```python
from build123d import *

# Parameters (mm, degrees)
SKETCH1_R           = 75
SKETCH1_R_2         = 1.7
SKETCH1_R_3         = 15
BOSS_EXTRUDE1_DEPTH = 3
SKETCH2_R           = 1.75
CUT_EXTRUDE2_DEPTH  = 107.108435103
SKETCH3_R           = 1.75
CUT_EXTRUDE3_DEPTH  = 107.108435103


with BuildPart() as part:
    # Sketch1 → Boss-Extrude1 (new body)
    with BuildSketch(Plane(origin=(0, 0, 0), x_dir=(1, 0, 0), z_dir=(0, 1, 0))):
        with Locations(Location((0, 0, 0), (0, 0, 270))):
            Circle(SKETCH1_R)
        with Locations(Location((49.497474683, 49.497474683, 0), (0, 0, 270))):
            Circle(SKETCH1_R_2, mode=Mode.SUBTRACT)
        with Locations(Location((-49.497474683, 49.497474683, 0), (0, 0, 270))):
            Circle(SKETCH1_R_2, mode=Mode.SUBTRACT)
        with Locations(Location((-49.497474683, -49.497474683, 0), (0, 0, 270))):
            Circle(SKETCH1_R_2, mode=Mode.SUBTRACT)
        with Locations(Location((49.497474683, -49.497474683, 0), (0, 0, 270))):
            Circle(SKETCH1_R_2, mode=Mode.SUBTRACT)
        with Locations(Location((0, 0, 0), (0, 0, 270))):
            Circle(SKETCH1_R_3, mode=Mode.SUBTRACT)
    extrude(amount=BOSS_EXTRUDE1_DEPTH)

    # Sketch2 → Cut-Extrude2 (cut, through all)
    with BuildSketch(Plane(origin=(0, 0, 0), x_dir=(1, 0, 0), z_dir=(0, 1, 0))):
        with Locations(Location((0, 68.825, 0), (0, 0, 270))):
            Circle(SKETCH2_R)
        with Locations(Location((68.825, 0, 0), (0, 0, 270))):
            Circle(SKETCH2_R)
        with Locations(Location((0, -68.825, 0), (0, 0, 270))):
            Circle(SKETCH2_R)
        with Locations(Location((-68.825, 0, 0), (0, 0, 270))):
            Circle(SKETCH2_R)
    extrude(amount=CUT_EXTRUDE2_DEPTH, mode=Mode.SUBTRACT)

    # Sketch3 → Cut-Extrude3 (cut, through all)
    with BuildSketch(Plane(origin=(0, 0, 0), x_dir=(1, 0, 0), z_dir=(0, 1, 0))):
        with Locations(Location((-43, 25, 0), (0, 0, 270))):
            Circle(SKETCH3_R)
        with Locations(Location((-17, 25, 0), (0, 0, 270))):
            Circle(SKETCH3_R)
        with Locations(Location((-17, -41, 0), (0, 0, 270))):
            Circle(SKETCH3_R)
        with Locations(Location((-43, -41, 0), (0, 0, 270))):
            Circle(SKETCH3_R)
        with Locations(Location((17.505557347, 19.884131141, 0), (0, 0, 270))):
            Circle(SKETCH3_R)
        with Locations(Location((46.494442653, -19.884131141, 0), (0, 0, 270))):
            Circle(SKETCH3_R)
        with Locations(Location((46.494442653, 19.884131141, 0), (0, 0, 270))):
            Circle(SKETCH3_R)
        with Locations(Location((17.505557347, -19.884131141, 0), (0, 0, 270))):
            Circle(SKETCH3_R)
        Polygon((31.243092686, 49.296238796), (12.765502036, 56.949907443), (14.678919198, 61.569305106), (33.156509848, 53.915636458), align=None)
    extrude(amount=CUT_EXTRUDE3_DEPTH, mode=Mode.SUBTRACT)


solid = part.part
```
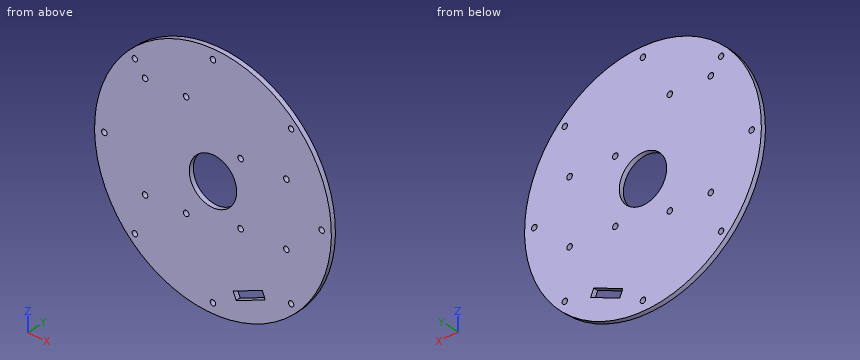
Source: CAD feature listing. Evaluate the final solid. Frame: model axes, mm. Give positions to 0.01 mm unless a question says otherwise; leave off trailing zeros. Write each loop counter-clockwise with the first axis right and the second up, starting at its lowest first coordinate (ties: lowest second). Pieces come first, ordered by that corner, then holes.
1. Section query D-D (z = 0). Return the cut outline in (x, y) (3 decimals), then the cut area to 3 significant figures.
2. Material intervals for line 1 along X through (y, z) = (1.7, 0) (3 decimals); line 2 along Z through (x, y) = (-1, 2.7); line 3 along Z through (x, y) = (50, 1.7), sorted ascending.
3. Section query B-B (z = -25). Return the cut outline in (x, y).
4. Section query A-A (x = 0). Return the cut outline in (y, z) (3 decimals).
5. First-contact query: pin 1 (3 mm diameter, centred on x = 0, z = -68.825, fed in from +Y); pin 2 (1 mm diameter, centred on x = -57, y = 1.5, fed in from +Z). Flat tips, straight axial feed; report the tip coordinate or a pass-through.
6. Section query C-C (y = 1.8). Count the separate pieces of the cut face and the enclosed holes in it, then the cut area to 3 significant figures.
Output values:
1. outline: (-75, 0) - (-70.575, 0) - (-70.575, 3) - (-75, 3) - close; (-67.075, 0) - (-15, 0) - (-15, 3) - (-67.075, 3) - close; (15, 0) - (67.075, 0) - (67.075, 3) - (15, 3) - close; (70.575, 0) - (75, 0) - (75, 3) - (70.575, 3) - close
1. area: 339 mm2
2. line 1: x = -75 to -70.575, -67.075 to -15, 15 to 67.075, 70.575 to 75
2. line 2: z = -74.99 to -70.26, -67.39 to -14.97, 14.97 to 67.39, 70.26 to 74.99
2. line 3: z = -55.9 to -51.12, -47.87 to 47.87, 51.12 to 55.9
3. outline: (-70.71, 0) - (-44.75, 0) - (-44.75, 3) - (-70.71, 3) - close; (-41.25, 0) - (-18.75, 0) - (-18.75, 3) - (-41.25, 3) - close; (-15.25, 0) - (70.71, 0) - (70.71, 3) - (-15.25, 3) - close
4. outline: (0, -75) - (3, -75) - (3, -70.575) - (0, -70.575) - close; (0, -67.075) - (3, -67.075) - (3, -15) - (0, -15) - close; (0, 15) - (3, 15) - (3, 67.075) - (0, 67.075) - close; (0, 70.575) - (3, 70.575) - (3, 75) - (0, 75) - close
5. pin 1: passes through
5. pin 2: stops at z = 49.32
6. separate pieces: 1
6. enclosed holes: 18
6. area: 16,700 mm2
